Answer from the drawing. Dimensions are ordinates in mm from the lowest x, y and z of the part. Coordinates: 2 decimals unless noted, no trailing zeros. Loops run counter-clockwise (first coordinate to the right, second up) from the corner with the lowest first, then second, coordinate; pieces in that order, holes last.
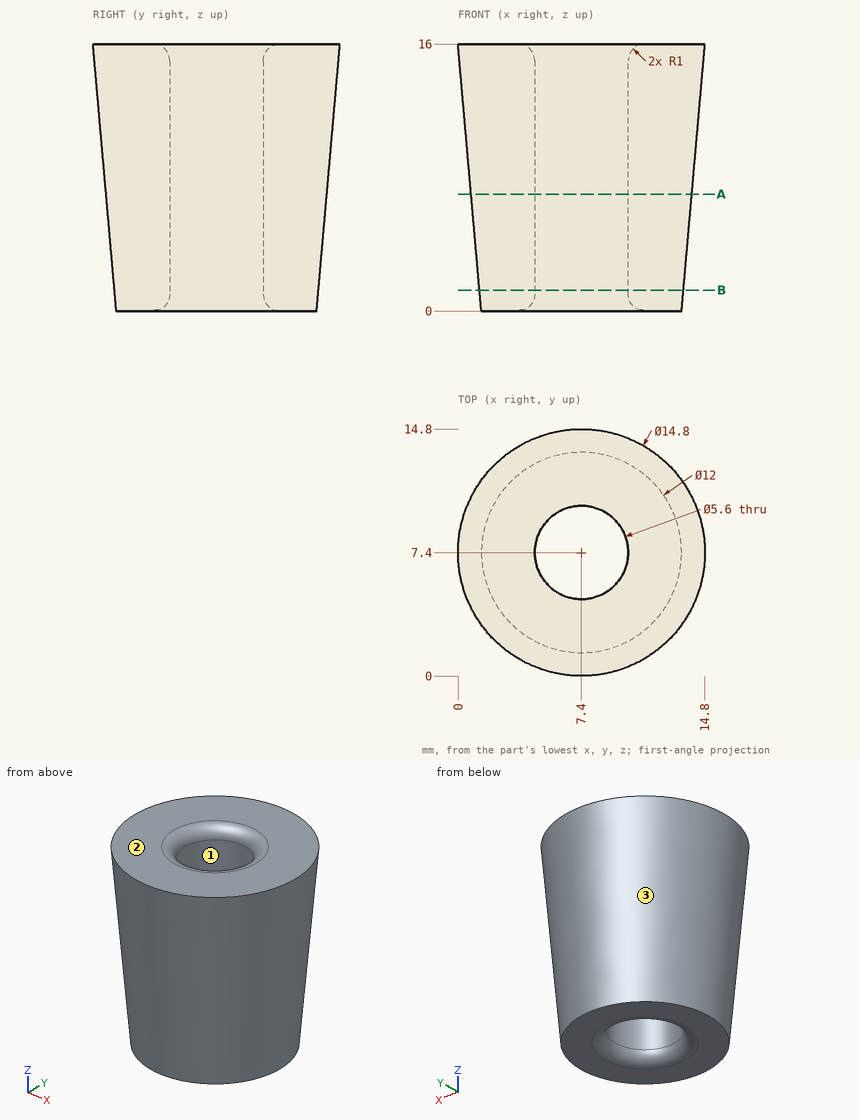
Item 1: A cutting plane is placed at A-A on z = 7. Determine the outline of the cut face in (x, y) (1 decimal), then the cut area to 3 significant figures.
Numbers:
outline: circle Ø13.2 at (7.4, 7.4); hole circle Ø5.6 at (7.4, 7.4)
area: 113 mm2
Item 2: Given pin 1 (5 mm diameter, centred on y = 9, z = 12, fed in from +X); pin 2 (6 mm diameter, centred on y = 7.5, z = 4.5, fed in from +X); pin 3 (1.5 mm diameter, centred on x = 8, z = 8.5, fed in from +Y), each flat-ended and moving along its own axis, determine where each tip first touches the part or whether it passes through.
Numbers:
pin 1: stops at x = 14.63
pin 2: stops at x = 14.06
pin 3: stops at y = 14.2
Item 3: Find the intervals of material crossed by line 1 along Y through (x, z) = (8.5, 7.25) (1 decimal); line 2 along X through (y, z) = (9.5, 8.5); line 3 along X through (y, z) = (6.75, 2.5) (1 decimal), in increasing order.
Numbers:
line 1: y = 0.9 to 4.8, 10 to 13.9
line 2: x = 0.99 to 5.55, 9.25 to 13.81
line 3: x = 1.2 to 4.7, 10.1 to 13.6
Item 4: A cutting plane is placed at B-B on z = 1.25. Determine the outline of the cut face in (x, y).
Numbers:
outline: circle Ø12.22 at (7.4, 7.4); hole circle Ø5.6 at (7.4, 7.4)
Item 5: Determine the mould class of the marked faces 1, 2 and 3 for opening direction X: released by +X, released by -X, zero draft, split by the parting line, or undercut.
Numbers:
face 1: undercut
face 2: zero draft
face 3: split by the parting line
